```python
from build123d import *

# Parameters (mm, degrees)
BOSS_EXTRUDE1_DEPTH = 1.5
SKETCH2_R           = 0.55
CUT_EXTRUDE1_DEPTH  = 1.5
SCALE1_SCALE        = 2.5


with BuildPart() as part:
    # Sketch1 → Boss-Extrude1 (new body)
    with BuildSketch(Plane(origin=(0, 0, 0), x_dir=(1, 0, 0), z_dir=(0, 1, 0))):
        with BuildLine():
            Line((58.878887557, 2), (78.578887557, 2))
            ThreePointArc((78.578887557, 2), (80.578887557, 0), (78.578887557, -2))
            Line((78.578887557, -2), (58.878887557, -2))
            ThreePointArc((58.878887557, -2), (56.878887557, 0), (58.878887557, 2))
        make_face()
    extrude(amount=BOSS_EXTRUDE1_DEPTH)

    # Sketch2 → Cut-Extrude1 (cut)
    with BuildSketch(Plane(origin=(0, 1.5, 0), x_dir=(1, 0, 0), z_dir=(0, 1, 0))):
        with Locations(Location((79.041953668, 0, 0), (0, 0, 270))):
            Circle(SKETCH2_R)
        with Locations(Location((76.541953668, 0, 0), (0, 0, 270))):
            Circle(SKETCH2_R)
        with Locations(Location((74.041953668, 0, 0), (0, 0, 270))):
            Circle(SKETCH2_R)
        with Locations(Location((71.541953668, 0, 0), (0, 0, 270))):
            Circle(SKETCH2_R)
        with Locations(Location((69.041953668, 0, 0), (0, 0, 270))):
            Circle(SKETCH2_R)
        with Locations(Location((66.541953668, 0, 0), (0, 0, 270))):
            Circle(SKETCH2_R)
        with Locations(Location((64.041953668, 0, 0), (0, 0, 270))):
            Circle(SKETCH2_R)
        with Locations(Location((61.541953668, 0, 0), (0, 0, 270))):
            Circle(SKETCH2_R)
    extrude(amount=-CUT_EXTRUDE1_DEPTH, mode=Mode.SUBTRACT)


with BuildPart() as part_1:
    # Scale1: scaled about (68.587018838, 0.75, 0)
    add(part.part.scale(SCALE1_SCALE).moved(Location((-102.880528257, -1.125, 0))))


solid = part_1.part
```
Geometry: final body of the model. Coordinates: model frame, mm. Coordinates: 2 decimals unless noted, no trailing zeros. Loops run counter-clockwise (first coordinate to the right, second up) from the corner with the lowest first, then second, coordinate; pieces in that order, holes last. Notation, with made-up numbers: (-16.75, -12.75) -> (10.25, -12.75) arc R10 ccw to (10.25, 5.25) -> close; hole circle Ø4 at (-2, -37.75). An arc over 180 degrees is marked (long way). Use a Markdown table: item, result. Add a question column.
(1) Line query: line 1 along Z through (x, y) = (94, 1); line 2 along Z through (x, y) = (95, 1.75); line 3 along Z through (x, y) = (44, 0.5). Output: solid intervals per line, ascending.
(2) Pin query (flat end, axial travel): pin 1 Ø2.5 at (x, z) = (94.72, 0) entering from -Y. Return the tip coordinate at first contact, or that it passes through.
(3) Section query C-C, the plane z = 4.5. Return loops of the section in (x, y) (3 decimals).
(4) Section query A-A, the plane y = 1.55. State how many separate pieces and enclosed holes the cut face has, plus the area to 3 significant figures.
(5) Section query D-D, the plane x = 43. Return loops of the section in (y, z) (3 decimals).
(6) Mould query, pull axis Z, two halves, no side actions, for faces 1 (the cylindrical face through (95.884, 0.776, 0.739)), 2 (the flat face through (69, -1.125, -2)), 3 (the flat face through (69, 1, -5)), 4 (the cylindrical face through (77.134, 0.776, 0.739)). Classes: pulls with the +Z half, pulls with the -Z half, needs draft (parallel to the pull), parting line crosses it, or undercut.
Answer:
| question | item | result |
|---|---|---|
| 1 | line 1 | z = -4.98 to -1.17, 1.17 to 4.98 |
| 1 | line 2 | z = -4.79 to -1.35, 1.35 to 4.79 |
| 1 | line 3 | z = -4.99 to 4.99 |
| 2 | pin 1 | passes through |
| 3 | outline | (42.137, -1.125) -> (95.746, -1.125) -> (95.746, 2.625) -> (42.137, 2.625) -> close |
| 4 | separate pieces | 1 |
| 4 | enclosed holes | 8 |
| 4 | area | 524 mm^2 |
| 5 | outline | (-1.125, -4.824) -> (2.625, -4.824) -> (2.625, 4.824) -> (-1.125, 4.824) -> close |
| 6 | face 1 | undercut |
| 6 | face 2 | needs draft |
| 6 | face 3 | pulls with the -Z half |
| 6 | face 4 | undercut |
